Can you work these out from the model? Positions are in its coordinate system, mm. Round coordinates to 2 decimals unless told otherwise and drop trailing zeros. Loops run counter-clockwise (first coordinate to the right, second up) from the corner with the lowest first, then second, coordinate; pieces in that order, holes last. Notation, with made-up numbers: M 89.25,-20.5 L 125.25,-20.5 A10 cw 125.25,-6.5 Z; hole C 85.25,-14 d10. An arc over 180 degrees is marked long. Return JSON: item names as keys, results as strings.
Autodesk Inventor part; units mm, degrees
ref_plane "YZ Plane" through (0, 0, 0) normal (1, 0, 0) x (0, 1, 0)
ref_plane "XZ Plane" through (0, 0, 0) normal (0, 1, 0) x (-1, 0, 0)
ref_plane "XY Plane" through (0, 0, 0) normal (0, 0, 1) x (1, 0, 0)
sketch "Sketch1" plane through (0, 0, 0) normal (0, 0, 1) x (1, 0, 0)
  line L0 (0, 0) -> (40, 0)
  line L1 (40, 0) -> (40, 20)
  line L2 (40, 20) -> (0, 20)
  line L3 (0, 20) -> (0, 0)
  point P0 (7.5, 10)
  point P1 (32.5, 10)
  point P2 (40, 10)
  dimension "d0" = 20
  dimension "d1" = 7.5
  dimension "d2" = 7.5
  dimension "d3" = 25
extrude "Extrusion1" add sketch "Sketch1" against normal blind 5
hole "Hole1" at (7.5, 10, 0) at (32.5, 10, 0) direction (0, 0, -1) diameter 3.2 depth 25.4 tip angle 118
fillet "Fillet1" radius 4 4 edges at (40, 20, -2.5) (40, 0, -2.5) (0, 0, -2.5) (0, 20, -2.5)
properties part number "Spacer"
Q1. Suppose I cut it at C-C, the plane z = -4.5. Please give me the cut outline in (x, y), plus the area to 3 significant figures.
Results:
{"outline": "M 0,4 A4 ccw 4,0 L 36,0 A4 ccw 40,4 L 40,16 A4 ccw 36,20 L 4,20 A4 ccw 0,16 Z; hole C 7.5,10 d3.2; hole C 32.5,10 d3.2", "area": "770 mm2"}
Q2. Suppose I cut it at B-B, the plane x = 32.5. Please give me the cut outline in (y, z), plus the area to 3 significant figures.
Results:
{"outline": "M 0,-5 L 8.4,-5 L 8.4,0 L 0,0 Z; M 11.6,-5 L 20,-5 L 20,0 L 11.6,0 Z", "area": "84.0 mm2"}
Q3. If I drill on line 1 along X through (y, z) = (10, -3.3); line 2 along Y through (x, z) = (32.5, -2.7); line 3 along X through (y, z) = (16.25, -2.4), over which ranges is the centre line in solid material (lowest first)?
Results:
{"line 1": "x = 0 to 5.9, 9.1 to 30.9, 34.1 to 40", "line 2": "y = 0 to 8.4, 11.6 to 20", "line 3": "x = 0.01 to 39.99"}
Q4. I'm going to push a flat-ended pin straight in: pin 1 Ø3 at (x, y) = (32.5, 10) entering from +Z (3 decimals). Where does the tip first touch, or does it pass through?
Results:
{"pin 1": "passes through"}
Q5. Suppose I cut it at D-D, the plane y = 17.75. Please give me the cut outline in (x, z), plus the area to 3 significant figures.
Results:
{"outline": "M 0.4,-5 L 39.6,-5 L 39.6,0 L 0.4,0 Z", "area": "196 mm2"}
Q6. Suppose I cut it at A-A, the plane y = 10. Please give me the cut outline in (x, z).
Results:
{"outline": "M 0,-5 L 5.9,-5 L 5.9,0 L 0,0 Z; M 9.1,-5 L 30.9,-5 L 30.9,0 L 9.1,0 Z; M 34.1,-5 L 40,-5 L 40,0 L 34.1,0 Z"}
Q7. Thinking about a two-plate mould opening in Y: for faces 1 (the cylindrical face through (38.859, 1.203, -2.535)), 2 (the cylindrical face through (8.47, 11.27, -2.54)), 3 (the cylindrical face through (33.47, 11.27, -2.54)), 4 (the flat face through (20, 10, -5)), which applies, pulls with the +Y half, pulls with the -Y half, needs draft (parallel to the pull), parting line crosses it, or undercut?
Results:
{"face 1": "pulls with the -Y half", "face 2": "undercut", "face 3": "undercut", "face 4": "needs draft"}
